Could you check a few things on this model? Use its own coordinates, in mm. Face numbers are marked on the shaded views. A direction names the side the tool comes from. Give positions to 0.01 mm unless a question says otherwise; leave off trailing zeros. Order: outer loops, then holes, each group sorted by start corner. A loop starts at its lowest first (then second) coordinate and runs counter-clockwise, first axis right, second up.
(1) If we mould it in two halves opening along X, with no side actions, what happens to the marked faces 3, 4 and 5? For each: released by +X, released by -X, zero draft, split by the parting line, or undercut.
(2) Imagine slicing it at D-D, the plane z = 55. Write out the boundary of the cut face in (x, y) (3 decimals), then the cut area to 3 significant figures.
(3) If I drill on probe 1 along Z at (x, y) = (-8, -30.5); probe 2 along X at (y, z) = (13, 57) (3 decimals); probe 3 along Z at (x, y) = (-46, -33.5), over which ranges is the centre line in solid material (lowest first)?
(4) On a 3-axis mill with a long thin cutter (end or side, diameter ignored), from which of +Z, -Z, +X, -X, +Y, -Y can I reach the whole of each face in a straight line? I mean the marked faces 1 and 2. Say none if no direction works.
(5) Imagine slicing it at B-B, the plane x = 0. Write out the boundary of the cut face in (y, z) (3 decimals).
(6) Imagine slicing it at A-A, the plane z = -126. Write out the boundary of the cut face in (x, y) (3 decimals).
(7) Imagine slicing it at C-C, the plane y = 17.5. Write out the boundary of the cut face in (x, z) (3 decimals), then the cut area to 3 significant figures.
(8) Will these pins go through, and if not, where does the flat tip stop? pin 1 (8 mm diameter, centred on x = 11.5, y = -19, fed in from -Z); pin 2 (10.5 mm diameter, centred on x = 33.5, z = 142.5, fed in from -Y) (3 decimals); pin 3 (6 mm diameter, centred on x = -41.5, y = -20, fed in from +Z); pin 4 (4.5 mm diameter, centred on y = 27.5, z = 143.5, fed in from +X).
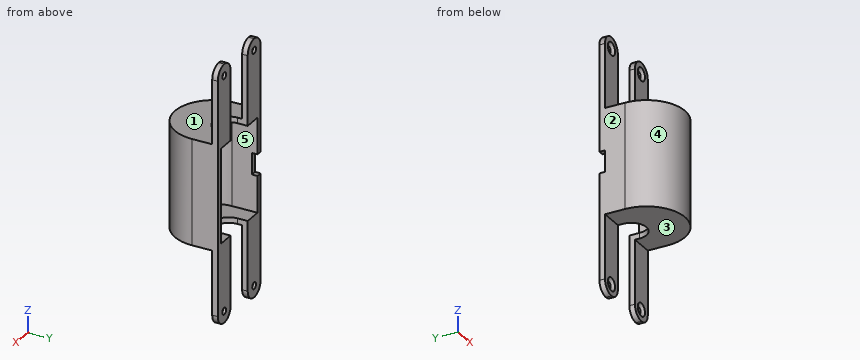
from build123d import *

# Parameters (mm, degrees)
BOSS_EXTRUDE2_DEPTH = 78.232
SHELL1_T            = -8.255
SKETCH2_W           = 31.75
SKETCH2_H           = 8.255
CUT_EXTRUDE1_DEPTH  = 8.255
SKETCH3_W           = 34.29
SKETCH3_H           = 8.255
BOSS_EXTRUDE3_DEPTH = 112.141
CUT_EXTRUDE2_START  = -8.255
CUT_EXTRUDE2_DEPTH  = 8.255


# Read off the part's stored shape, not the designer's step: Cut-Extrude2
with BuildPart() as part:
    # Sketch1 → Boss-Extrude2 (new, symmetric)
    with BuildSketch(Plane.XY):
        with BuildLine():
            Line((22.86, 38.1), (57.15, 38.1))
            Line((57.15, 38.1), (57.15, 0))
            ThreePointArc((57.15, 0), (0, -57.15), (-57.15, 0))
            Line((-57.15, 0), (-57.15, 38.1))
            Line((-57.15, 38.1), (-22.86, 38.1))
            Line((-22.86, 38.1), (-22.86, 22.86))
            ThreePointArc((-22.86, 22.86), (0, 0), (22.86, 22.86))
            Line((22.86, 22.86), (22.86, 38.1))
        make_face()
    extrude(amount=BOSS_EXTRUDE2_DEPTH, both=True)

    # Shell1
    shell1_openings = [part.faces().sort_by_distance(p)[0] for p in [
        (40.005, 38.1, 0),
        (-40.005, 38.1, 0),
        (-22.86, 30.48, 0),
        (0, 0, 0),
        (22.86, 30.48, 0),
    ]]
    offset(amount=SHELL1_T, openings=shell1_openings, kind=Kind.INTERSECTION)

    # Sketch2 → Cut-Extrude1 (cut)
    with BuildSketch(Plane(origin=(-48.895, 0, 0), x_dir=(0, 0, -1), z_dir=(1, 0, 0))):
        with Locations((0, 33.9725)):
            Rectangle(SKETCH2_W, SKETCH2_H)
    extrude(amount=-CUT_EXTRUDE1_DEPTH, mode=Mode.SUBTRACT)


with BuildPart() as body_2:
    # Sketch3 → Boss-Extrude3 (new body)
    with BuildSketch(Plane.XY.offset(78.232)):
        with Locations((-40.005, 33.9725)):
            Rectangle(SKETCH3_W, SKETCH3_H)
    extrude(amount=BOSS_EXTRUDE3_DEPTH)

    # Cut-Extrude2 outline → Cut-Extrude2 (cut)
    with BuildSketch(Plane(origin=(0, 38.1, 0), x_dir=(1, 0, 0), z_dir=(0, 1, 0)).offset(CUT_EXTRUDE2_START)):
        with BuildLine():
            Line((-22.86, -190.373), (-22.86, -173.228))
            ThreePointArc((-22.86, -173.228), (-27.881654237, -185.351345763), (-40.005, -190.373))
            Line((-40.005, -190.373), (-22.86, -190.373))
        make_face()
        with BuildLine():
            Line((-57.15, -190.373), (-40.005, -190.373))
            ThreePointArc((-40.005, -190.373), (-52.128345763, -185.351345763), (-57.15, -173.228))
            Line((-57.15, -173.228), (-57.15, -190.373))
        make_face()
    extrude(amount=CUT_EXTRUDE2_DEPTH, mode=Mode.SUBTRACT)

    # Sketch7 → CSK for 3/8 Flat Head Machine Screw (100)1 (revolve, cut)
    with BuildSketch(Plane(origin=(-40.005, 29.845, 173.228), x_dir=(0, 0, -1), z_dir=(1, 0, 0))):
        Polygon((0, 0), (0, 8.255), (5.0419, 8.255), (5.0419, 3.88964634), (9.6774, 0), align=None)
    revolve(axis=Axis((-40.005, 23.495, 173.228), (0, 1, 0)), mode=Mode.SUBTRACT)


with BuildPart() as body_3:
    # Mirror2: mirrored copy
    add(body_2.part.mirror(Plane(origin=(0, 0, 0), x_dir=(0, 0, 1), z_dir=(1, 0, 0))))


with BuildPart() as body_4:
    # Mirror3: mirrored copy
    add(body_2.part.mirror(Plane.XY))


with BuildPart() as body_5:
    # Mirror3 2: mirrored copy
    add(body_3.part.mirror(Plane.XY))


with BuildPart() as body_2_1:
    add(body_2.part)

    # Combine2: union body 3, body 4, body 5, part
    add(body_3.part)
    add(body_4.part)
    add(body_5.part)
    add(part.part)


solid = body_2_1.part
Answer block:
1. face 3: zero draft
1. face 4: split by the parting line
1. face 5: undercut
2. outline: (-57.15, 0) arc R57.15 ccw to (57.15, 0) - (57.15, 38.1) - (48.895, 38.1) - (48.895, 0) arc R48.895 cw to (-48.895, 0) - (-48.895, 38.1) - (-57.15, 38.1) - close
2. area: 2,000 mm2
3. probe 1: z = -78.23 to -69.98, 69.98 to 78.23
3. probe 2: x = -57.15 to -48.895, 48.895 to 57.15
3. probe 3: z = -78.23 to 78.23
4. face 1: +Z, +X, -X, -Y
4. face 2: +Z, -Z, -X, +Y, -Y
5. outline: (-57.15, -78.232) - (0, -78.232) - (0, -69.977) - (-48.895, -69.977) - (-48.895, 69.977) - (0, 69.977) - (0, 78.232) - (-57.15, 78.232) - close
6. outline: (-57.15, 29.845) - (-22.86, 29.845) - (-22.86, 38.1) - (-57.15, 38.1) - close; (22.86, 29.845) - (57.15, 29.845) - (57.15, 38.1) - (22.86, 38.1) - close
7. outline: (-57.15, -78.232) - (-22.223, -78.232) - (-22.223, -69.977) - (-48.895, -69.977) - (-48.895, 69.977) - (-22.223, 69.977) - (-22.223, 78.232) - (-57.15, 78.232) - close; (22.223, -78.232) - (57.15, -78.232) - (57.15, 78.232) - (22.223, 78.232) - (22.223, 69.977) - (48.895, 69.977) - (48.895, -69.977) - (22.223, -69.977) - close
7. area: 3,460 mm2
8. pin 1: stops at z = -78.23
8. pin 2: stops at y = 29.845
8. pin 3: stops at z = 78.23
8. pin 4: passes through
